The model under review builds one solid part; all positions refer to its coordinate system, in mm. Face numbers are marked on the shaded views. A direction names the side the tool comes from. Coordinates: 2 decimals unless noted, no trailing zeros. Loops run counter-clockwise (first coordinate to the right, second up) from the corner with the lowest first, then second, coordinate; pieces in that order, holes last. Notation, with made-up numbers: M 30.25,45 L 49.25,45 A13 ccw 49.25,50 Z; hole C 37.5,31 d4. An arc over 180 degrees is marked long. Use one line per item in the form item = value.
Autodesk Fusion 360 part; units mm, degrees
sketch "Sketch1" plane through (0, 0, 0) normal (1, 0, 0) x (0, 1, 0) in component "Wing"
  line L0 (0, 0) -> (31.75, 0)
  line L1 (31.75, 0) -> (31.75, 44.45)
  line L2 (31.75, 44.45) -> (0, 44.45)
  line L3 (0, 44.45) -> (0, 0)
  dimension "d1" = 31.75
  dimension "d2" = 44.45
extrude "Extrude1" add sketch "Sketch1" against normal blind 5 makes body 1 in component "Wing"
sketch "Sketch3" plane through (-5, 0, 0) normal (-1, 0, 0) x (0, -1, 0) in component "Wing"
  line L0 (0, 0) -> (0, 44.45)
  line L1 (0, 44.45) -> (-31.75, 44.45)
  line L2 (-31.75, 44.45) -> (-31.75, 0)
  line L3 (-31.75, 0) -> (0, 0)
  line L4 (-25.497, 41.8155) -> (-18.997, 41.8155)
  line L5 (-18.997, 41.8155) -> (-18.997, 35.3155)
  line L6 (-18.997, 35.3155) -> (-25.497, 35.3155)
  line L7 (-25.497, 35.3155) -> (-25.497, 41.8155)
  circle A0 centre (-18.997, 38.5655) radius 3.25
  circle A1 centre (-25.497, 38.5655) radius 3.25
  dimension "d13" = 6.5
  dimension "d14" = 6.5
  dimension "d15" = 6.5
  dimension "d16" = 6.5
extrude "Extrude2" add sketch "Sketch3" against normal blind 5 separate body contours L7 A1 | L4 A0 A1 | L7 A1 | L5 A0 | L5 A0 | L6 A0 A1 makes body 2 in component "Wing"
copy_body "CopyPasteBodies1" bodies 2 makes body 3 in component "Wing"
move_body "Move1" bodies 3 to x (1, 0, 0) y (0, 1, 0) z (0, 0, 1) at (0, 0, -35.25) in component "Wing"
move_body "Move2" bodies 3 to x (1, 0, 0) y (0, 1, 0) z (0, 0, 1) at (0, 0, 2.8) in component "Wing"
combine "Combine1" operation cut target body 1 tool bodies 2 3 in component "Wing"
component "Wing" placed x (1, 0, 0) y (0, 1, 0) z (0, 0, 1) at (0, 0, 0)
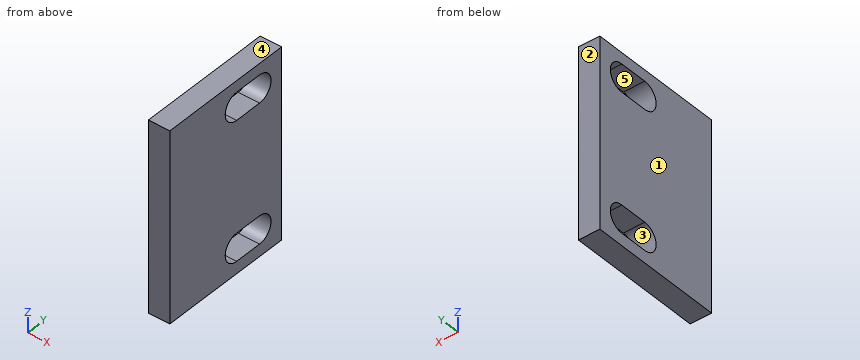
1. Machinability: for the marked faces 4 and 5, which of the approach directions +Z, -Z, +X, -X, +Y, -Y give a long, thin tool a straight path to every point of the face, cutting with its end or side? Answer none if there is none.
Response values:
face_4 = +Z, +X, -X, +Y, -Y
face_5 = +X, -X
2. Wall thickness on line 1 along Z through (x, y) = (-3.1, 25.5); line 2 along Y through (x, z) = (-1.8, 7); line 3 along Y through (x, z) = (-0.7, 8.5): over which ranges is each line inside the solid? List them lowest first. Write a range as from..to.
Response values:
line_1 = 0..2.87, 9.37..35.32, 41.82..44.45
line_2 = 0..15.87, 28.62..31.75
line_3 = 0..16.79, 27.71..31.75
3. Add section D-D (y = 27.5). State the section outline as (x, z) points.
Response values:
outline = M -5,0 L 0,0 L 0,3.56 L -5,3.56 Z; M -5,8.67 L 0,8.67 L 0,36.01 L -5,36.01 Z; M -5,41.12 L 0,41.12 L 0,44.45 L -5,44.45 Z
4. The part is to be moulded in two halves that separate along Y. For the marked faces 1, 2 and 3, say which applies: pulls with the +Y half, pulls with the -Y half, needs draft (parallel to the pull), parting line crosses it, or undercut.
Response values:
face_1 = needs draft
face_2 = pulls with the +Y half
face_3 = undercut
5. Add section C-C (z = 38.5). State the section outline as (x, y) points, then the cut area to 3 significant figures.
Response values:
outline = M -5,0 L 0,0 L 0,15.75 L -5,15.75 Z; M -5,28.75 L 0,28.75 L 0,31.75 L -5,31.75 Z
area = 93.8 mm^2
6. Add section B-B (y = 20.5). State the section outline as (x, z) points, then the cut area to 3 significant figures.
Response values:
outline = M -5,0 L 0,0 L 0,2.87 L -5,2.87 Z; M -5,9.37 L 0,9.37 L 0,35.32 L -5,35.32 Z; M -5,41.82 L 0,41.82 L 0,44.45 L -5,44.45 Z
area = 157 mm^2
7. Add section A-A (x = -3.85). State the section outline as (y, z) points, then the cut area to 3 significant figures.
Response values:
outline = M 0,0 L 31.75,0 L 31.75,44.45 L 0,44.45 Z; hole M 19,2.87 L 25.5,2.87 A3.25 ccw 25.5,9.37 L 19,9.37 A3.25 ccw Z; hole M 19,35.32 L 25.5,35.32 A3.25 ccw 25.5,41.82 L 19,41.82 A3.25 ccw Z
area = 1,260 mm^2
